```python
from build123d import *

# Parameters (mm, degrees)
F0_W          = 165
F0_H          = 314
F0_W_2        = 157
F0_H_2        = 306
F1_DEPTH      = 50
F3_DEPTH      = 90
F4_R          = 5
F5_DEPTH      = 14
F5_DEPTH_BACK = 70
F6_DEPTH      = 50
F7_W          = 4
F7_H          = 58
F8_DEPTH      = 300
F9_W          = 58
F9_H          = 4
F10_DEPTH     = 345
F11_W         = 314
F11_H         = 4
F12_DEPTH     = 90
F13_W         = 4
F13_H         = 314
F14_DEPTH     = 300
F15_R         = 5
F16_DEPTH     = 29


# Not quite as in the source:
# - a feature names something its author has since deleted; it is built from what else it names


with BuildPart() as f1:
    # F0 (on Top) → F1 (new body)
    with BuildSketch(Plane.XY):
        with Locations((0, -8.0325696617)):
            Rectangle(F0_W, F0_H)
        with Locations((0, -8.0325696617)):
            Rectangle(F0_W_2, F0_H_2, mode=Mode.SUBTRACT)
    extrude(amount=F1_DEPTH)

    # F2 (on face) → F3 (join)
    with BuildSketch(Plane(origin=(-82.5, 0, 0), x_dir=(0, -1, 0), z_dir=(-1, 0, 0))):
        Polygon((36.0325696617, 0), (65.0325696617, 0), (65.0325696617, 4), (40.0325696617, 4), (40.0325696617, 46), (65.0325696617, 46), (65.0325696617, 50), (36.0325696617, 50), align=None)
        Polygon((65.0325696617, 4), (65.0325696617, 0), (94.0325696617, 0), (94.0325696617, 50), (65.0325696617, 50), (65.0325696617, 46), (90.0325696617, 46), (90.0325696617, 4), align=None)
    extrude(amount=F3_DEPTH)

    # F4 (on face) → F5 (cut, two sides)
    with BuildSketch(Plane.XY.offset(4)) as f5_sk:
        with Locations((-92.5, -65.0325696617)):
            Circle(F4_R)
        with Locations((-162.5, -65.0325696617)):
            Circle(F4_R)
    extrude(amount=-F5_DEPTH, mode=Mode.SUBTRACT)
    extrude(f5_sk.sketch, amount=F5_DEPTH_BACK, mode=Mode.SUBTRACT)

    # F4 (on face) → F6 (cut)
    with BuildSketch(Plane.XY.offset(4)):
        with Locations((-127.5, -65.0325696617)):
            Circle(F4_R)
    extrude(amount=F6_DEPTH, mode=Mode.SUBTRACT)

    # F7 (on face) → F8 (join)
    with BuildSketch(Plane(origin=(0, 0, 0), x_dir=(1, 0, 0), z_dir=(0, 0, -1))):
        with Locations((-174.5, 65.0325696617)):
            Rectangle(F7_W, F7_H)
    extrude(amount=-F8_DEPTH)

    # F9 (on face) → F10 (join)
    with BuildSketch(Plane.YZ.offset(-172.5)):
        with Locations((-65.0325696617, 298)):
            Rectangle(F9_W, F9_H)
    extrude(amount=F10_DEPTH)

    # F11 (on face) → F12 (join)
    with BuildSketch(Plane.YZ.offset(82.5)):
        with Locations((-8.0325696617, 2)):
            Rectangle(F11_W, F11_H)
    extrude(amount=F12_DEPTH)

    # F13 (on face) → F14 (join)
    with BuildSketch(Plane(origin=(0, 0, 0), x_dir=(1, 0, 0), z_dir=(0, 0, -1))):
        with Locations((174.5, 8.0325696617)):
            Rectangle(F13_W, F13_H)
    extrude(amount=-F14_DEPTH)

    # F15 (on face) → F16 (cut)
    with BuildSketch(Plane.XY.offset(300)):
        with Locations((-92.5, -69.0325696617)):
            Circle(F15_R)
        with Locations((-127.5, -69.0325696617)):
            Circle(F15_R)
        with Locations((-162.5, -69.0325696617)):
            Circle(F15_R)
    extrude(amount=-F16_DEPTH, mode=Mode.SUBTRACT)


solid = f1.part
```
Geometry check sheet. Reference: the model listing, model coordinates, mm. A direction names the side the tool comes from. Round coordinates to 2 decimals unless told otherwise and drop trailing zeros. Order: outer loops, then holes, each group sorted by start corner. A loop starts at its lowest first (then second) coordinate and runs counter-clockwise, first axis right, second up. Notation, with made-up numbers: (6, 66.25) - (43, 66.25) arc R17 cw to (43, 89.25) - close; hole circle Ø5 at (13.25, 65.5). An arc over 180 degrees is marked (long way). Use a Markdown table: item, result. Add a question column.
(1) Sectioned sample at D-D, the plane y = 14. Enter the section's corners in (x, z).
(2) Sectioned sample at B-B, the plane x = 0. Enter the section's corners in (y, z), and give its area (3 significant figures).
(3) Tool access check on faces 1 (the flat face through (-127, -90.033, 25)), 2 (the flat face through (-121, -65, 50)), 3 (the cylindrical face through (-166.47, -68.07, 47.97)). Record the directions out of +Z, -Z, +X, -X, +Y, -Y that give a thin tool (end or side, any length) a straight path to the whole face; none if there is none.
(4) Release check for a two-part mould opening along X. For faces 4 (the flat face through (-127, -40.033, 25)), 5 (the flat face through (115, -10, 0)), 6 (the flat face through (-176.5, -65, 148)) record: pulls with the +X half, pulls with the -X half, needs draft (parallel to the pull), parting line crosses it, or undercut.
(5) Depth check by flat-ended pin: pin 1 (6 mm diameter, centred on x = -162.5, y = -65.03, fed in from -Z); pin 2 (10 mm diameter, centred on y = 20, z = 173.5, fed in from -X); pin 3 (9 mm diameter, centred on x = -92.5, y = -65.03, fed in from +Z). Enter the tip coordinate at first touch or a pass-through.
(6) Sectioned sample at A-A, the plane z = 29.5. Enter the section's corners in (x, y), and give its area (3 significant figures).
(7) Sectioned sample at C-C, the plane z = 255. Enter the section's corners in (x, y).
(8) Material ranges on line 1 along Y through (x, z) = (-162.5, 2.65); line 2 along X through (y, z) = (-63, 96.5); line 3 along Y through (x, z) = (-92, 298), recorded low to high. Write a range as [from, to].
Answers below:
| question | item | result |
|---|---|---|
| 1 | outline | (-82.5, 0) - (-78.5, 0) - (-78.5, 50) - (-82.5, 50) - close; (78.5, 0) - (176.5, 0) - (176.5, 300) - (172.5, 300) - (172.5, 4) - (82.5, 4) - (82.5, 50) - (78.5, 50) - close |
| 2 | outline | (-165.03, 0) - (-161.03, 0) - (-161.03, 50) - (-165.03, 50) - close; (-94.03, 296) - (-36.03, 296) - (-36.03, 300) - (-94.03, 300) - close; (144.97, 0) - (148.97, 0) - (148.97, 50) - (144.97, 50) - close |
| 2 | area | 632 mm² |
| 3 | face 1 | none |
| 3 | face 2 | +Y, -Y |
| 3 | face 3 | -Z |
| 4 | face 4 | undercut |
| 4 | face 5 | needs draft |
| 4 | face 6 | pulls with the -X half |
| 5 | pin 1 | z = 296 |
| 5 | pin 2 | x = 172.5 |
| 5 | pin 3 | z = 300 |
| 6 | outline | (-176.5, -94.03) - (-82.5, -94.03) - (-82.5, -165.03) - (82.5, -165.03) - (82.5, 148.97) - (-82.5, 148.97) - (-82.5, -36.03) - (-176.5, -36.03) - close; (172.5, -165.03) - (176.5, -165.03) - (176.5, 148.97) - (172.5, 148.97) - close; hole (-172.5, -90.03) - (-82.5, -90.03) - (-82.5, -40.03) - (-172.5, -40.03) - close; hole (-78.5, -161.03) - (78.5, -161.03) - (78.5, 144.97) - (-78.5, 144.97) - close |
| 6 | area | 5,980 mm² |
| 7 | outline | (-176.5, -94.03) - (-172.5, -94.03) - (-172.5, -36.03) - (-176.5, -36.03) - close; (172.5, -165.03) - (176.5, -165.03) - (176.5, 148.97) - (172.5, 148.97) - close |
| 8 | line 1 | [-94.03, -70.03], [-60.03, -36.03] |
| 8 | line 2 | [-176.5, -172.5], [172.5, 176.5] |
| 8 | line 3 | [-94.03, -74.01], [-64.06, -36.03] |
